Build history of the part. All positions in model axes, mm. Face numbers are marked on the shaded views. A direction names the side the tool comes from. Round coordinates to 2 decimals unless told otherwise and drop trailing zeros. Write each loop counter-clockwise with the first axis right and the second up, starting at its lowest first coordinate (ties: lowest second). Pieces come first, ordered by that corner, then holes. Notation, with made-up numbers: (49, -38) - (76, -38) arc R8 cw to (76, -24) - close; hole circle Ø10 at (-9.75, 50). An arc over 180 degrees is marked (long way). Write each question's results on one line, items separated by ' | '.
Autodesk Inventor part; units mm, degrees
ref_plane "Work Plane2" through (-27, 9, 0) normal (1, 0, 0) x (0, 1, 0)
ref_plane "XY Plane" through (0, 0, 0) normal (0, 0, 1) x (1, 0, 0)
sketch "Sketch3" plane through (0, 0, 0) normal (1, 0, 0) x (0, 1, 0)
  line L0 (63.5252, 0) -> (0, 0) construction
  line L1 (0, -8) -> (0, -27)
  line L2 (0, -27) -> (18, -27)
  line L3 (18, -27) -> (18, -12.4)
  line L4 (9, -8) -> (9, -12.4)
  line L5 (9, -12.4) -> (18, -12.4)
  line L6 (9, -8) -> (5, -8)
  line L7 (5, -8) -> (5, 0)
  line L8 (0, -8) -> (0, 0)
  line L9 (5, 0) -> (0, 0)
  dimension "d15" = 18
  dimension "d18" = 9
  dimension "d32" = 27
  dimension "d33" = 12.4
  dimension "d54" = 4
  dimension "d56" = 8
revolve "Revolution1" add sketch "Sketch3" angle 360 about axis through (0, 63.5252, 0) along (0, -1, 0)
fillet "Fillet2" radius 1 2 edges at (0, 18, 27) (0, 0, 27)
ref_plane "Work Plane2" through (-27, 9, 0) normal (1, 0, 0) x (0, 1, 0)
sketch "Sketch4" plane through (-27, 9, 0) normal (1, 0, 0) x (0, 1, 0)
  line L0 (-9, 0) -> (10.8256, 0) construction
  line L1 (-3.75, 3.75) -> (3.75, 3.75)
  line L2 (3.75, 3.75) -> (3.75, -3.75)
  line L3 (3.75, -3.75) -> (-3.75, -3.75)
  line L4 (-3.75, -3.75) -> (-3.75, 3.75)
  line L5 (-3.75, 3.75) -> (3.75, -3.75) construction
  line L6 (3.75, 3.75) -> (-3.75, -3.75) construction
  line L7 (9, 26) -> (9, -26)
  point P0 (0, 0)
  dimension "d21" = 7.5
  dimension "d22" = 7.5
  dimension "d55" = 9
extrude "Extrusion3" cut sketch "Sketch4" along normal blind 10
pattern_circular "Circular Pattern2" count 3 over 360 about axis through (0, 13.5, 0) along (0, -1, 0) of "Extrusion3"
sketch "Sketch9" plane through (0, 18, 0) normal (0, 1, 0) x (1, 0, 0)
  circle A0 centre (0, -22.4737) radius 3.5
  point P0 (0, 0)
  dimension "d57" = 7
extrude "Extrusion7" cut sketch "Sketch9" against normal blind 2.4
ref_plane "Work Plane4" through (0, 9, 0) normal (0, 1, 0) x (-1, 0, 0)
split "Split1" plane through (0, 9, 0) removes the side toward (0, 1, 0)
properties part number "BasePaletasTop"
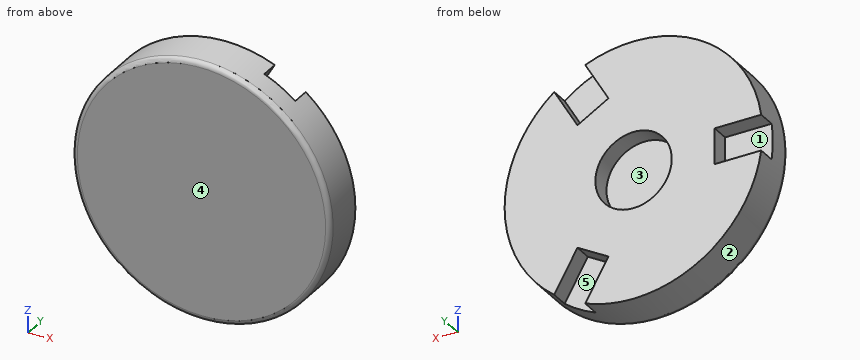
(1) Slice it at B-B, the plane x = 0. Write the cut outline in (y, z).
Worked answers:
outline: (0, -26) arc R1 ccw to (1, -27) - (9, -27) - (9, -8) - (5, -8) - (5, 8) - (9, 8) - (9, 27) - (1, 27) arc R1 ccw to (0, 26) - close
(2) Flat gauge pins, fed straight in: pin 1 Ø1.5 at (x, y) = (-4, 6) entering from -Z; pin 2 Ø3 at (x, y) = (-23, 6.5) entering from +Z; pin 3 Ø1.1 at (x, y) = (-23.5, 6.5) entering from -Z. Where does each tip first touch, or does it go through?
Worked answers:
pin 1: stops at z = -26.8 | pin 2: stops at z = 16.33 | pin 3: stops at z = -14.22
(3) Drill centre lines: probe 1 along X at (y, z) = (6.7, 0); probe 2 along Y at (x, z) = (10, -23.5); probe 3 along Z at (x, y) = (5, 7.5) (3 decimals). Where is each one in solid material? Low to high. Write a range as [from, to].
Worked answers:
probe 1: x = [-17, -8], [8, 27] | probe 2: y = [0, 5.25] | probe 3: z = [-26.533, -6.245], [6.245, 26.533]
(4) Two-plate mould, pull along X, no slides. Class the marked faces 1, 2 and 3: released by +X, released by -X, zero draft, split by the parting line, or undercut.
Worked answers:
face 1: zero draft | face 2: split by the parting line | face 3: undercut
(5) Slice it at C-C, the plane y = 3.75. Write the cut outline in (x, z).
Worked answers:
outline: circle Ø54 at (0, 0)
(6) Tool access for the marked faces 4 and 5: list every direction of +Z, -Z, +X, -X, +Y, -Y with a clear straight run to the whole face (end or side of a thin tool).
Worked answers:
face 4: +Z, -Z, +X, -X, -Y | face 5: +Y
(7) Slice it at A-A, the plane z = 0. Write the cut outline in (x, y), and give its area (3 significant figures).
Worked answers:
outline: (-27, 1) arc R1 ccw to (-26, 0) - (26, 0) arc R1 ccw to (27, 1) - (27, 9) - (8, 9) - (8, 5) - (-8, 5) - (-8, 9) - (-17, 9) - (-17, 5.25) - (-27, 5.25) - close | area: 384 mm2
